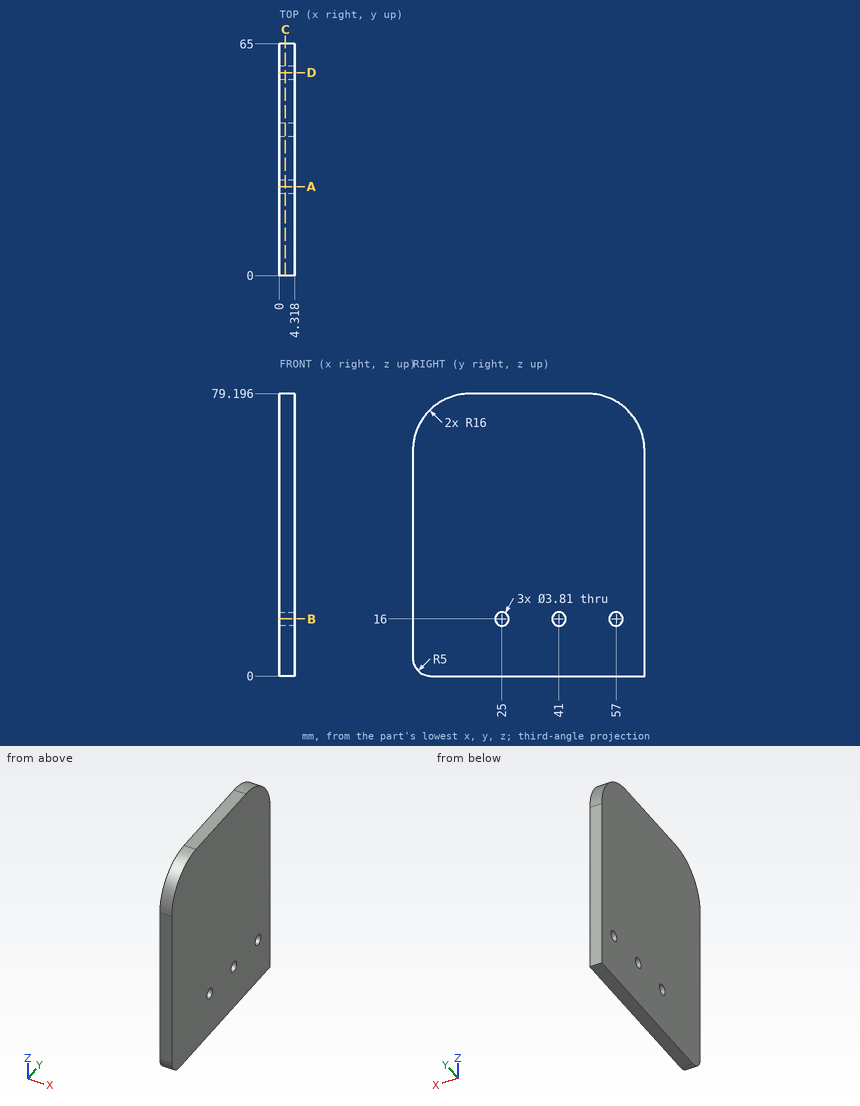
Could you check a few things on this drawing? It's one solid part, dimensions in mm from its lowest x, y, z. Coordinates: 2 decimals unless noted, no trailing zeros. Write each loop counter-clockwise with the first axis right and the second up, starting at its lowest first coordinate (ties: lowest second). Pieces come first, ordered by that corner, then holes. Notation, with made-up numbers: M 30,81 L 63,81 A8 ccw 63,95 Z; hole C -26.75,60.5 d1. An arc over 180 degrees is marked long. One line per question, with ' | ' between items.
1) Imagine slicing it at A-A, the plane y = 25. Write out the boundary of the cut face in (x, z) (3 decimals).
Checks:
outline: M 0,0 L 4.318,0 L 4.318,14.095 L 0,14.095 Z; M 0,17.905 L 4.318,17.905 L 4.318,79.196 L 0,79.196 Z
2) For pin 1 Ø2 at (x, y) = (3, 55.5) entering from +Z; pin 2 Ø3 at (y, z) = (57, 16) entering from -X, each with a flat end and sliding along its axis, tell me the tip position at first contact or that it passes through.
Checks:
pin 1: z = 78.22 | pin 2: through
3) Imagine slicing it at B-B, the plane z = 16. Write out the boundary of the cut face in (x, y) (3 decimals).
Checks:
outline: M 0,0 L 4.318,0 L 4.318,23.095 L 0,23.095 Z; M 0,26.905 L 4.318,26.905 L 4.318,39.095 L 0,39.095 Z; M 0,42.905 L 4.318,42.905 L 4.318,55.095 L 0,55.095 Z; M 0,58.905 L 4.318,58.905 L 4.318,65 L 0,65 Z
4) Imagine slicing it at C-C, the plane x = 1.65. Write out the boundary of the cut face in (y, z) (3 decimals).
Checks:
outline: M 0,5 A5 ccw 5,0 L 65,0 L 65,63.196 A16 ccw 49,79.196 L 16,79.196 A16 ccw 0,63.196 Z; hole C 25,16 d3.81; hole C 41,16 d3.81; hole C 57,16 d3.81
5) Imagine slicing it at D-D, the plane y = 57. Write out the boundary of the cut face in (x, z) (3 decimals), and give its area (3 significant figures).
Checks:
outline: M 0,0 L 4.318,0 L 4.318,14.095 L 0,14.095 Z; M 0,17.905 L 4.318,17.905 L 4.318,77.052 L 0,77.052 Z | area: 316 mm²
6) I need wall thicknesses on probe 1 along Y at (x, z) = (2.35, 16) (3 decimals); probe 2 along Z at (x, y) = (3.2, 26); probe 3 along Z at (x, y) = (0.55, 52). Which ranges of each line are inside material? Lowest first, please. Write a range as [from, to].
Checks:
probe 1: [0, 23.095], [26.905, 39.095], [42.905, 55.095], [58.905, 65] | probe 2: [0, 14.38], [17.62, 79.2] | probe 3: [0, 78.91]
